The model under review builds one solid part; all positions refer to its coordinate system, in mm. A direction names the side the tool comes from. Round coordinates to 2 decimals unless told otherwise and drop trailing zeros. Write each loop counter-clockwise with the first axis right and the second up, starting at its lowest first coordinate (ties: lowest second). Pieces come first, ordered by that corner, then holes. Notation, with made-up numbers: (82.5, 77.5) - (110.5, 77.5) arc R30 ccw to (110.5, 102.5) - close; hole circle Ø11 at (13.25, 34). An arc over 180 degrees is marked (long way). One line per question, with ' | ' between items. Start each with the question number.
```python
from build123d import *

# Parameters (mm, degrees)
SKETCH_1_W      = 50
SKETCH_1_H      = 25
SKETCH_1_R      = 2
SKETCH_1_R_2    = 0.9
EXTRUDE_1_DEPTH = 20
SHELL_1_T       = -1.5
SKETCH_1_3_R    = 2
SKETCH_1_3_R_2  = 0.9
EXTRUDE_2_DEPTH = 20


with BuildPart() as part:
    # Sketch 1 → Extrude 1 (new body)
    # profile 1 of 9: a face of its own
    with BuildSketch(Plane(origin=(0, 0, 0), x_dir=(1, 0, 0), z_dir=(0, 1, 0))):
        with Locations((25, 12.5)):
            Rectangle(SKETCH_1_W, SKETCH_1_H)
        with Locations((2.5, 2.5)):
            Circle(SKETCH_1_R, mode=Mode.SUBTRACT)
        with Locations((47.5, 2.5)):
            Circle(SKETCH_1_R, mode=Mode.SUBTRACT)
        with Locations((47.5, 22.5)):
            Circle(SKETCH_1_R, mode=Mode.SUBTRACT)
        with Locations((2.5, 22.5)):
            Circle(SKETCH_1_R, mode=Mode.SUBTRACT)
    # profile 2 of 9: a face of its own
    with BuildSketch(Plane(origin=(0, 0, 0), x_dir=(1, 0, 0), z_dir=(0, 1, 0))):
        with Locations((47.5, 2.5)):
            Circle(SKETCH_1_R)
        with Locations((47.5, 2.5)):
            Circle(SKETCH_1_R_2, mode=Mode.SUBTRACT)
    # profile 3 of 9: a face of its own
    with BuildSketch(Plane(origin=(0, 0, 0), x_dir=(1, 0, 0), z_dir=(0, 1, 0))):
        with Locations((47.5, 2.5)):
            Circle(SKETCH_1_R_2)
    # profile 4 of 9: a face of its own
    with BuildSketch(Plane(origin=(0, 0, 0), x_dir=(1, 0, 0), z_dir=(0, 1, 0))):
        with Locations((47.5, 22.5)):
            Circle(SKETCH_1_R)
        with Locations((47.5, 22.5)):
            Circle(SKETCH_1_R_2, mode=Mode.SUBTRACT)
    # profile 5 of 9: a face of its own
    with BuildSketch(Plane(origin=(0, 0, 0), x_dir=(1, 0, 0), z_dir=(0, 1, 0))):
        with Locations((47.5, 22.5)):
            Circle(SKETCH_1_R_2)
    # profile 6 of 9: a face of its own
    with BuildSketch(Plane(origin=(0, 0, 0), x_dir=(1, 0, 0), z_dir=(0, 1, 0))):
        with Locations((2.5, 2.5)):
            Circle(SKETCH_1_R)
        with Locations((2.5, 2.5)):
            Circle(SKETCH_1_R_2, mode=Mode.SUBTRACT)
    # profile 7 of 9: a face of its own
    with BuildSketch(Plane(origin=(0, 0, 0), x_dir=(1, 0, 0), z_dir=(0, 1, 0))):
        with Locations((2.5, 2.5)):
            Circle(SKETCH_1_R_2)
    # profile 8 of 9: a face of its own
    with BuildSketch(Plane(origin=(0, 0, 0), x_dir=(1, 0, 0), z_dir=(0, 1, 0))):
        with Locations((2.5, 22.5)):
            Circle(SKETCH_1_R)
        with Locations((2.5, 22.5)):
            Circle(SKETCH_1_R_2, mode=Mode.SUBTRACT)
    # profile 9 of 9: a face of its own
    with BuildSketch(Plane(origin=(0, 0, 0), x_dir=(1, 0, 0), z_dir=(0, 1, 0))):
        with Locations((2.5, 22.5)):
            Circle(SKETCH_1_R_2)
    extrude(amount=EXTRUDE_1_DEPTH)

    # Shell 1
    shell_1_openings = [part.faces().sort_by_distance(p)[0] for p in [
        (25, 20, -12.5),
    ]]
    offset(amount=SHELL_1_T, openings=shell_1_openings, kind=Kind.INTERSECTION)

    # Sketch 1_3 → Extrude 2 (add)
    # profile 1 of 4: a face of its own
    with BuildSketch(Plane(origin=(0, 0, 0), x_dir=(1, 0, 0), z_dir=(0, 1, 0))):
        with Locations((2.5, 22.5)):
            Circle(SKETCH_1_3_R)
        with Locations(Location((2.5, 22.5, 0), (0, 0, 270))):
            Circle(SKETCH_1_3_R_2, mode=Mode.SUBTRACT)
    # profile 2 of 4: a face of its own
    with BuildSketch(Plane(origin=(0, 0, 0), x_dir=(1, 0, 0), z_dir=(0, 1, 0))):
        with Locations((47.5, 22.5)):
            Circle(SKETCH_1_3_R)
        with Locations(Location((47.5, 22.5, 0), (0, 0, 270))):
            Circle(SKETCH_1_3_R_2, mode=Mode.SUBTRACT)
    # profile 3 of 4: a face of its own
    with BuildSketch(Plane(origin=(0, 0, 0), x_dir=(1, 0, 0), z_dir=(0, 1, 0))):
        with Locations((47.5, 2.5)):
            Circle(SKETCH_1_3_R)
        with Locations(Location((47.5, 2.5, 0), (0, 0, 270))):
            Circle(SKETCH_1_3_R_2, mode=Mode.SUBTRACT)
    # profile 4 of 4: a face of its own
    with BuildSketch(Plane(origin=(0, 0, 0), x_dir=(1, 0, 0), z_dir=(0, 1, 0))):
        with Locations((2.5, 2.5)):
            Circle(SKETCH_1_3_R)
        with Locations(Location((2.5, 2.5, 0), (0, 0, 270))):
            Circle(SKETCH_1_3_R_2, mode=Mode.SUBTRACT)
    extrude(amount=EXTRUDE_2_DEPTH)


solid = part.part
```
1. Add section A-A, the plane y = 2. Write out the cut boundary in (x, z).
2. Clearance check with a flat-ended pin moving along its axis: P1, Ø0.5, axis at x = 2, z = -2.5, coming from the +Y side. State where the tip first meets the part, or that it passes through.
3. Add section D-D, the plane x = 2.5. Write out the cut boundary in (y, z), then the cut area to 3 significant figures.
4. Wall thickness on line 1 along Z through (x, y) = (47.5, 8.25); line 2 along X through (y, z) = (9, -22.5); line 3 along Z through (x, y) = (31, 14.5): over which ranges is each line inside the solid? List them lowest first. Write a range as [from, to].
5. The part is to be moulded in two halves that separate along Z. For faces 3 (the face through (25, 0, -13)), 4 (the face through (1.5, 11, -12)), 5 (the face through (25, 10, -25)), say which applies: pulls with the +Z half, pulls with the -Z half, needs draft (parallel to the pull), parting line crosses it, or undercut.
6. Add section B-B, the plane z = -22.5. Write out the cut boundary in (x, y).
7. Add section C-C, the plane x = 44. Write out the cut boundary in (y, z), then the cut area to 3 significant figures.
8. Machinability: for faces 1 (the face through (0, 10, -12)), 2 (the face through (1.702, 10.62, -22.085)), which of the approach directions +Z, -Z, +X, -X, +Y, -Y give a long, thin tool a straight path to every point of the face, cutting with its end or side? Answer none if there is none.
Geometry check:
1) outline: (0, -25) - (50, -25) - (50, 0) - (0, 0) - close; hole (1.5, -20.77) arc R2 cw to (4.23, -23.5) - (45.77, -23.5) arc R2 cw to (48.5, -20.77) - (48.5, -4.23) arc R2 cw to (45.77, -1.5) - (4.23, -1.5) arc R2 cw to (1.5, -4.23) - close; hole circle Ø1.8 at (2.5, -22.5); hole circle Ø1.8 at (2.5, -2.5); hole circle Ø1.8 at (47.5, -22.5); hole circle Ø1.8 at (47.5, -2.5)
2) P1: stops at y = 1.5
3) outline: (0, -25) - (20, -25) - (20, -23.4) - (1.5, -23.4) - (1.5, -21.6) - (20, -21.6) - (20, -20.5) - (1.5, -20.5) - (1.5, -4.5) - (20, -4.5) - (20, -3.4) - (1.5, -3.4) - (1.5, -1.6) - (20, -1.6) - (20, 0) - (0, 0) - close | area: 137 mm2
4) line 1: z = [-25, -23.4], [-21.6, -20.5], [-4.5, -3.4], [-1.6, 0] | line 2: x = [0, 1.6], [3.4, 4.5], [45.5, 46.6], [48.4, 50] | line 3: z = [-25, -23.5], [-1.5, 0]
5) face 3: needs draft | face 4: undercut | face 5: pulls with the -Z half
6) outline: (0, 0) - (50, 0) - (50, 20) - (48.4, 20) - (48.4, 1.5) - (46.6, 1.5) - (46.6, 20) - (45.5, 20) - (45.5, 1.5) - (4.5, 1.5) - (4.5, 20) - (3.4, 20) - (3.4, 1.5) - (1.6, 1.5) - (1.6, 20) - (0, 20) - close
7) outline: (0, -25) - (20, -25) - (20, -23.5) - (1.5, -23.5) - (1.5, -1.5) - (20, -1.5) - (20, 0) - (0, 0) - close | area: 93.0 mm2
8) face 1: +Z, -Z, -X, +Y, -Y | face 2: +Y
